Autodesk Inventor part; units mm, degrees
ref_plane "YZ Plane" through (0, 0, 0) normal (1, 0, 0) x (0, 1, 0)
ref_plane "XZ Plane" through (0, 0, 0) normal (0, 1, 0) x (-1, 0, 0)
ref_plane "XY Plane" through (0, 0, 0) normal (0, 0, 1) x (1, 0, 0)
sketch "Sketch1" plane through (0, 0, 0) normal (0, 1, 0) x (-1, 0, 0)
  line L0 (-50, 25) -> (50, 25)
  line L1 (50, 25) -> (50, -25)
  line L2 (50, -25) -> (-50, -25)
  line L3 (-50, -25) -> (-50, 25)
  line L4 (-50, 25) -> (0, 25)
  line L5 (0, 25) -> (0, 75)
  line L6 (0, 75) -> (-50, 75)
  line L7 (-50, 75) -> (-50, 25)
  line L8 (50, -25) -> (40, -25)
  line L9 (40, -25) -> (40, -15)
  line L10 (-50, -25) -> (-50, -15)
  line L11 (-50, -15) -> (-40, -15)
  circle A0 centre (40, -15) radius 4
  circle A1 centre (-40, -15) radius 4
  point P0 (0, 0)
  point P1 (0, 25)
  dimension "d0" = 100
  dimension "d1" = 50
  dimension "d2" = 50
  dimension "d3" = 50
  dimension "d4" = 10
  dimension "d5" = 10
  dimension "d6" = 10
  dimension "d7" = 10
  dimension "d8" = 8
  dimension "d9" = 8
  dimension "d12" = 90
  dimension "d13" = 90
extrude "Extrusion1" add sketch "Sketch1" along normal blind 2
properties part number "Pinz"
Geometry: final body of the model. Coordinates: model frame, mm. Coordinates: 2 decimals unless noted, no trailing zeros. Write each loop counter-clockwise with the first axis right and the second up, starting at its lowest first coordinate (ties: lowest second). Pieces come first, ordered by that corner, then holes. Notation, with made-up numbers: M -29.75,82 L -25.75,82 A15 ccw -25.75,107 Z; hole C 16.25,46 d7. An arc over 180 degrees is marked long. Answer as CSV lines item,"result". Start each with the question number.
Q1. Cut plane C-C on z = -15. Return the cut outline in (x, y).
Q2. Cut plane D-D on x = 40. Return the cut outline in (y, z), then the cut area to 3 significant figures.
Q3. Cut plane A-A on x = -40. Return the cut outline in (y, z), then the cut area to 3 significant figures.
Q4. Cut plane B-B on y = 1.4. Return the cut outline in (x, z), then the cut area to 3 significant figures.
Q5. Line query: line 1 (Z direction, x = 40, y = 1.3); line 2 (Z direction, x = -40, y = 0.8); line 3 (X direction, y = 0.9, z = -13.5). Output: solid intervals per line, ascending. Write a range as from..to.
Q6. Mould query, pull axis X, two halves, no side actions, for faces 1 (the flat face through (12, 0, 15)), 2 (the cylindrical face through (42.95, 0.99, -17.7)). Classes: released by +X, released by -X, zero draft, split by the parting line, or undercut.
Findings below:
1,outline,"M -50,0 L -44,0 L -44,2 L -50,2 Z; M -36,0 L 36,0 L 36,2 L -36,2 Z; M 44,0 L 50,0 L 50,2 L 44,2 Z"
2,outline,"M 0,-25 L 2,-25 L 2,-19 L 0,-19 Z; M 0,-11 L 2,-11 L 2,75 L 0,75 Z"
2,area,"184 mm2"
3,outline,"M 0,-25 L 2,-25 L 2,-19 L 0,-19 Z; M 0,-11 L 2,-11 L 2,25 L 0,25 Z"
3,area,"84.0 mm2"
4,outline,"M -50,-25 L 50,-25 L 50,75 L 0,75 L 0,25 L -50,25 Z; hole C -40,-15 d8; hole C 40,-15 d8"
4,area,"7,400 mm2"
5,line 1,"z = -25..-19, -11..75"
5,line 2,"z = -25..-19, -11..25"
5,line 3,"x = -50..-43.71, -36.29..36.29, 43.71..50"
6,face 1,"zero draft"
6,face 2,"undercut"
